Build history of the part. All positions in model axes, mm. Face numbers are marked on the shaded views. Round coordinates to 2 decimals unless told otherwise and drop trailing zeros. Loops run counter-clockwise (first coordinate to the right, second up) from the corner with the lowest first, then second, coordinate; pieces in that order, holes last. Notation, with made-up numbers: (-18.5, 55) -> (18.5, 55) arc R25 ccw to (18.5, 84) -> close; hole circle Ø5 at (62.25, 88.25). An arc over 180 degrees is marked (long way). Put each result on its own line as item: value. Start each with the question number.
Item 1: Cut at A-A, the plane y = -16. List the corners of the cut face in (x, z), plus the area to 3 significant figures.
Item 2: Drill centre lines: probe 1 along Z at (x, y) = (0, -17.75); probe 2 along Z at (x, y) = (44, -7); probe 3 along X at (y, z) = (-16.75, -67.5). Where is each one in solid material? Low to high. Write a range as [from, to].
Item 3: Flat gauge pins, fed straight in: pin 1 Ø5 at (y, z) = (-21, -15) entering from -X; pin 2 Ø12 at (y, z) = (-8, -9) entering from +X; pin 3 Ø5 at (y, z) = (-16.5, 20) entering from +X. Where does each tip first touch, or does it go through?
Item 4: Pull direction Z, two halves, no side cores. Call the marked faces 1 and 2: +Z half, -Z half, draft (parallel to the pull), parting line (faces both ways), or undercut.
```python
from build123d import *

# Parameters (mm, degrees)
F1_DEPTH = 25.4
F2_R     = 90.4905202305
F3_DEPTH = 25.4
F4_R     = 5.08
F5_R     = 5.08


with BuildPart() as f1:
    # F0 (on Front) → F1 (new body)
    with BuildSketch(Plane.XZ):
        Polygon((108.2512310565, 103.2173403296), (71.7572271824, 124.2871632902), (35.2632233082, 145.3569862507), (-48.9206086824, 141.3468160806), (-117.5724930729, 92.4600305138), (-148.8959416402, 14.2178385502), (-132.9459807853, -68.5384166946), (-74.7866103824, -129.5342089082), (7.1169803999, -149.4038050384), (86.7609801915, -121.8387487058), (138.858981796, -55.5907505305), (146.870237811, 28.3069181527), align=None)
        Polygon((-16.0764054761, 73.5763918309), (71.7572271824, 124.2871632902), (71.7572271824, 25.0510078709), (72.8934520967, 23.3153364586), (71.7572271824, 0), (71.7572271824, -124.2871632902), (-143.5144543648, 0), (-52.9619502577, 52.280512622), (-41.3737298926, 66.6985122387), align=None, mode=Mode.SUBTRACT)
        Polygon((71.7572271824, -124.2871632902), (71.7572271824, 0), (70.6210022681, -23.3153364586), (41.3737298926, -59.7046308119), (-3.6769010605, -71.953072985), (-47.3230807818, -55.3821743769), (-72.8934520967, -16.3214550319), (-70.6210022681, 30.3092178854), (-52.9619502577, 52.280512622), (-143.5144543648, 0), align=None)
        Polygon((71.7572271824, 25.0510078709), (71.7572271824, 124.2871632902), (-16.0764054761, 73.5763918309), (3.6769010605, 78.9469544117), (47.3230807818, 62.3760558037), align=None)
        Polygon((-52.9619502577, 52.280512622), (-16.0764054761, 73.5763918309), (-41.3737298926, 66.6985122387), align=None)
    extrude(amount=F1_DEPTH)

    # F2 (on face) → F3 (cut)
    with BuildSketch(Plane.XZ.offset(25.4)):
        Circle(F2_R)
        Polygon((72.8934520967, 23.3153364586), (70.6210022681, -23.3153364586), (41.3737298926, -59.7046308119), (-3.6769010605, -71.953072985), (-47.3230807818, -55.3821743769), (-72.8934520967, -16.3214550319), (-70.6210022681, 30.3092178854), (-52.9619502577, 52.280512622), (-16.0764054761, 73.5763918309), (3.6769010605, 78.9469544117), (47.3230807818, 62.3760558037), align=None, mode=Mode.SUBTRACT)
    extrude(amount=-F3_DEPTH, mode=Mode.SUBTRACT)

    # F4
    f4_edges = [f1.edges().sort_by_distance(p)[0] for p in [
        (-133.234217, -25.4, 53.338935),
        (-140.920961, -25.4, -27.160289),
        (-103.866296, -25.4, -99.036313),
        (-33.834815, -25.4, -139.469007),
        (46.93898, -25.4, -135.621277),
        (112.809981, -25.4, -88.71475),
        (142.86461, -25.4, -13.641916),
        (127.560734, -25.4, 65.762129),
        (71.757227, -25.4, 124.287163),
        (-6.828693, -25.4, 143.351901),
        (-83.246551, -25.4, 116.903423),
    ]]
    fillet(f4_edges, radius=F4_R)

    # F5
    f5_edges = [f1.edges().sort_by_distance(p)[0] for p in [
        (127.560734, 0, 65.762129),
        (142.86461, 0, -13.641916),
        (112.809981, 0, -88.71475),
        (46.93898, 0, -135.621277),
        (-33.834815, 0, -139.469007),
        (-103.866296, 0, -99.036313),
        (-140.920961, 0, -27.160289),
        (-6.828693, 0, 143.351901),
        (71.757227, 0, 124.287163),
        (-83.246551, 0, 116.903423),
        (-133.234217, 0, 53.338935),
    ]]
    fillet(f5_edges, radius=F5_R)


solid = f1.part
```
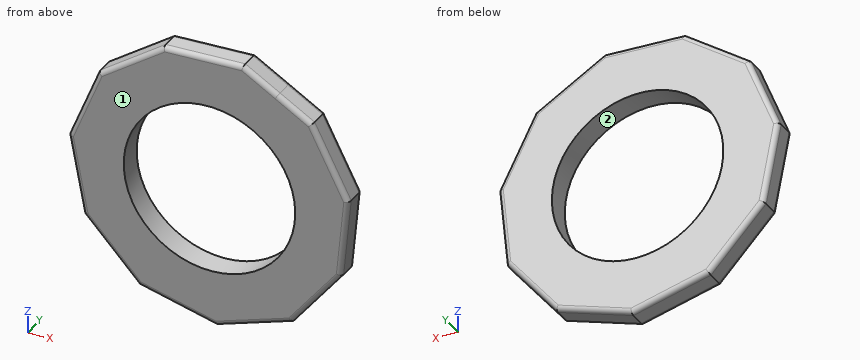
Reply:
1. outline: (-148.9, 14.22) -> (-132.95, -68.54) -> (-74.79, -129.53) -> (7.12, -149.4) -> (86.76, -121.84) -> (138.86, -55.59) -> (146.87, 28.31) -> (108.25, 103.22) -> (35.26, 145.36) -> (-48.92, 141.35) -> (-117.57, 92.46) -> close; hole circle Ø180.98 at (0, 0)
1. area: 40,800 mm^2
2. probe 1: z = [-147.68, -90.49], [90.49, 143.68]
2. probe 2: z = [-136.64, -79.07], [79.07, 140.31]
2. probe 3: x = [-133.15, -60.27], [60.27, 129.49]
3. pin 1: stops at x = -143.73
3. pin 2: stops at x = 143.88
3. pin 3: stops at x = 146.32
4. face 1: draft
4. face 2: undercut
